Here's how the part is built. I have some questions about the finished solid (model axes, mm). A direction names the side the tool comes from. Coordinates: 2 decimals unless noted, no trailing zeros. Write each loop counter-clockwise with the first axis right and the second up, starting at its lowest first coordinate (ties: lowest second). Pieces come first, ordered by that corner, then holes. Notation, with made-up numbers: (33.25, 55.5) -> (89.25, 55.5) arc R23 cw to (89.25, 70.5) -> close; hole circle Ø5 at (62.25, 76). An arc over 180 degrees is marked (long way). Put each result on its own line as item: value. Start each with the question number.
Item 1: On a 3-axis mill with a long thin cutter (end or side, diameter ignored), from which of +Z, -Z, +X, -X, +Y, -Y can I reach the whole of each face in a straight line? I mean faces 1 (the face through (43, -1, 25)), 2 (the face through (-1, -36, 17)), 3 (the face through (-1, 38, 25)). Say none if no direction works.
Item 2: I want a section at D-D, the plane x = -29.5. List the corners of the cut face in (y, z) for me.
Item 3: If we mould it in two halves opening along X, with no side actions, what happens to faces 4 (the face through (-1, 1, 0)), 5 (the face through (-36.028, -41.972, 7.43)), 6 (the face through (-43, -1, 25)), 7 (the face through (-41, -1, 17))? For each: released by +X, released by -X, zero draft, split by the parting line, or undercut.
Item 4: I need wall thicknesses on line 1 (Y direction, x = -14, z = 19.75); line 2 (X direction, y = -12, z = 25.5); line 3 (X direction, y = 23, z = 17). Which ranges of each line are inside material? Lowest first, please. Write a range as [from, to].
Item 5: I want a section at A-A, the plane y = -32. List the corners of the cut face in (x, z) for me, then the cut area to 3 significant figures.
Item 6: I want a section at C-C, the plane y = 4.5. List the corners of the cut face in (x, z) for me.
Item 7: For pin 1 (1.5 mm diameter, centred on x = 16.5, z = 22, fed in from -Y); pin 2 (5 mm diameter, centred on x = 11.5, z = 24, fed in from +Y); pin 3 (6 mm diameter, centred on x = 30.5, y = -23.5, fed in from +Z), each with a flat end and sliding along its axis, tell me the tip position at first contact or that it passes through.
Item 8: I want a section at B-B, the plane z = 23.5. List the corners of the cut face in (x, y) for me, then the cut area to 3 significant figures.
from build123d import *

# Parameters (mm, degrees)
SKETCH1_W                     = 90
SKETCH1_H                     = 80
BOSS_EXTRUDE1_DEPTH           = 30
SHELL1_T                      = -4
SKETCH4_W                     = 7
SKETCH4_H                     = 10
BOSS_EXTRUDE2_DEPTH           = 4
BOSS_EXTRUDE2_DRAFT           = 15
BOSS_EXTRUDE2_PROFILE_2_DEPTH = 4
BOSS_EXTRUDE2_PROFILE_2_DRAFT = 15
SKETCH6_R                     = 3
CUT_EXTRUDE3_DEPTH            = 10
SKETCH8_W                     = 90
SKETCH8_H                     = 80
SKETCH8_W_2                   = 86
SKETCH8_H_2                   = 76
CUT_EXTRUDE4_DEPTH            = 10


with BuildPart() as part:
    # Sketch1 → Boss-Extrude1 (new body)
    with BuildSketch(Plane.XY):
        Rectangle(SKETCH1_W, SKETCH1_H)
    extrude(amount=BOSS_EXTRUDE1_DEPTH)

    # Shell1
    shell1_openings = [part.faces().sort_by_distance(p)[0] for p in [
        (0, 0, 30),
    ]]
    offset(amount=SHELL1_T, openings=shell1_openings, kind=Kind.INTERSECTION)


with BuildPart() as boss_extrude2_tool:
    # Sketch4 → Boss-Extrude2 (with draft: the straight prism first)
    with BuildSketch(Plane.XZ.offset(40)):
        with Locations((-39, 7.5)):
            Rectangle(SKETCH4_W, SKETCH4_H)
    extrude(amount=BOSS_EXTRUDE2_DEPTH)
    # Boss-Extrude2: the draft: its side faces are tilted about the plane it starts from
    boss_extrude2_sides = [boss_extrude2_tool.faces().sort_by_distance(p)[0] for p in [
        (-42.5, -42, 7.5),
        (-39, -42, 2.5),
        (-35.5, -42, 7.5),
        (-39, -42, 12.5),
    ]]
    draft(boss_extrude2_sides, Plane.XZ.offset(40), BOSS_EXTRUDE2_DRAFT)


with BuildPart() as part_1:
    add(part.part)

    # Boss-Extrude2: add boss_extrude2_tool
    add(boss_extrude2_tool.part)


with BuildPart() as boss_extrude2_profile_2_tool:
    # Sketch4 → Boss-Extrude2 profile 2 (with draft: the straight prism first)
    with BuildSketch(Plane.XZ.offset(40)):
        with Locations((39, 7.5)):
            Rectangle(SKETCH4_W, SKETCH4_H)
    extrude(amount=BOSS_EXTRUDE2_PROFILE_2_DEPTH)
    # Boss-Extrude2 profile 2: the draft: its side faces are tilted about the plane it starts from
    boss_extrude2_profile_2_sides = [boss_extrude2_profile_2_tool.faces().sort_by_distance(p)[0] for p in [
        (35.5, -42, 7.5),
        (39, -42, 2.5),
        (42.5, -42, 7.5),
        (39, -42, 12.5),
    ]]
    draft(boss_extrude2_profile_2_sides, Plane.XZ.offset(40), BOSS_EXTRUDE2_PROFILE_2_DRAFT)


with BuildPart() as part_2:
    add(part_1.part)

    # Boss-Extrude2 profile 2: add boss_extrude2_profile_2_tool
    add(boss_extrude2_profile_2_tool.part)

    # Sketch6 → Cut-Extrude3 (cut)
    with BuildSketch(Plane.XY.offset(4)):
        with Locations((-37, -32)):
            Circle(SKETCH6_R)
    extrude(amount=-CUT_EXTRUDE3_DEPTH, mode=Mode.SUBTRACT)

    # Sketch8 → Cut-Extrude4 (cut)
    with BuildSketch(Plane.XY.offset(30)):
        Rectangle(SKETCH8_W, SKETCH8_H)
        Rectangle(SKETCH8_W_2, SKETCH8_H_2, mode=Mode.SUBTRACT)
    extrude(amount=-CUT_EXTRUDE4_DEPTH, mode=Mode.SUBTRACT)


solid = part_2.part
Calculated:
1. face 1: +Z, +X, +Y, -Y
1. face 2: +Z
1. face 3: +Z, +X, -X, +Y
2. outline: (-40, 0) -> (40, 0) -> (40, 20) -> (38, 20) -> (38, 30) -> (36, 30) -> (36, 4) -> (-36, 4) -> (-36, 30) -> (-38, 30) -> (-38, 20) -> (-40, 20) -> close
3. face 4: zero draft
3. face 5: undercut
3. face 6: released by -X
3. face 7: undercut
4. line 1: y = [-40, -36], [36, 40]
4. line 2: x = [-43, -41], [41, 43]
4. line 3: x = [-45, -41], [41, 45]
5. outline: (-45, 0) -> (-40, 0) -> (-40, 4) -> (-41, 4) -> (-41, 30) -> (-43, 30) -> (-43, 20) -> (-45, 20) -> close; (-34, 0) -> (45, 0) -> (45, 20) -> (43, 20) -> (43, 30) -> (41, 30) -> (41, 4) -> (-34, 4) -> close
5. area: 504 mm2
6. outline: (-45, 0) -> (45, 0) -> (45, 20) -> (43, 20) -> (43, 30) -> (41, 30) -> (41, 4) -> (-41, 4) -> (-41, 30) -> (-43, 30) -> (-43, 20) -> (-45, 20) -> close
7. pin 1: stops at y = -38
7. pin 2: stops at y = 38
7. pin 3: stops at z = 4
8. outline: (-43, -38) -> (43, -38) -> (43, 38) -> (-43, 38) -> close; hole (-41, -36) -> (41, -36) -> (41, 36) -> (-41, 36) -> close
8. area: 632 mm2
